Build history of the part. All positions in model axes, mm. Give positions to 0.01 mm unless a question says otherwise; leave off trailing zeros. Write each loop counter-clockwise with the first axis right and the second up, starting at its lowest first coordinate (ties: lowest second). Pieces come first, ordered by that corner, then holes. Notation, with made-up numbers: (30.5, 59) -> (85.5, 59) arc R21 ccw to (85.5, 71) -> close; hole circle Ø3 at (78.25, 39.5). An arc over 180 degrees is marked (long way). Put each result on its own line as item: value. Start each with the question number.
Item 1: Flat gauge pins, fed straight in: pin 1 Ø1.5 at (y, z) = (-53, 2) entering from -X; pin 2 Ø1 at (y, z) = (-55, 2) entering from -X. Where does each tip first touch, or does it go through?
Item 2: Slice it at B-B, the plane z = 2.3. List the corners of the cut face in (x, y).
Item 3: Slice it at C-C, the plane y = -68. List the corners of the cut face in (x, z).
Item 4: Drill centre lines: line 1 along X through (y, z) = (-64.5, 1.9); line 2 along X through (y, z) = (-65.5, 1.25); line 3 along Y through (x, z) = (70, 1.1). Where is each one in solid material? Low to high.
Item 5: Slice it at A-A, the plane x = 76. List the corners of the cut face in (y, z), plus the area to 3 significant figures.
Item 6: Slice it at D-D, the plane y = -35.5. List the corners of the cut face in (x, z), plus the area to 3 significant figures.
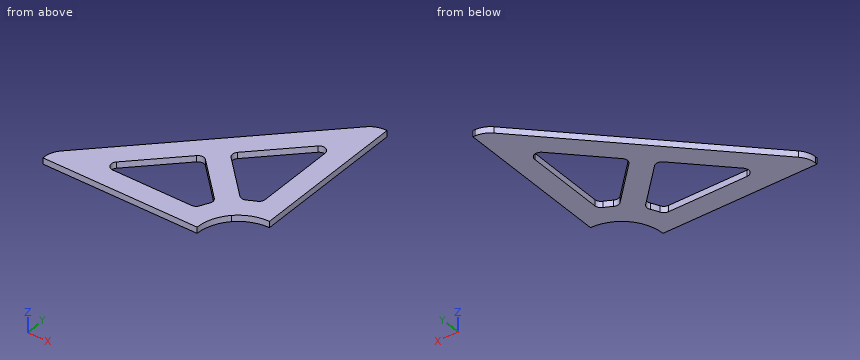
```python
from build123d import *

# Parameters (mm, degrees)
F1_DEPTH = 3
F2_R     = 3
F3_W     = 5
F3_H     = 3
F4_DEPTH = 25
F5_W     = 5
F5_H     = 3
F6_DEPTH = 25
F7_R     = 10


with BuildPart() as f1:
    # F0 (on Top) → F1 (new body)
    with BuildSketch(Plane.XY):
        with BuildLine():
            Line((50, -50), (0, -100))
            Line((0, -100), (70, -100))
            ThreePointArc((70, -100), (70.4320432104, -94.9269406382), (71.7157287525, -90))
            Line((71.7157287525, -90), (24.1421356237, -90))
            Line((24.1421356237, -90), (53.5355339059, -60.6066017178))
            Line((53.5355339059, -60.6066017178), (75.5479654307, -82.6190332426))
            ThreePointArc((75.5479654307, -82.6190332426), (77.0871215252, -80.635083269), (78.7867965644, -78.7867965644))
            Line((78.7867965644, -78.7867965644), (50, -50))
        make_face()
        with BuildLine():
            ThreePointArc((71.7157287525, -90), (70.4320432104, -94.9269406382), (70, -100))
            Line((70, -100), (80, -100))
            ThreePointArc((80, -100), (81.5224093498, -92.3463313527), (85.8578643763, -85.8578643763))
            Line((85.8578643763, -85.8578643763), (78.7867965644, -78.7867965644))
            ThreePointArc((78.7867965644, -78.7867965644), (77.0871215252, -80.635083269), (75.5479654307, -82.6190332426))
            ThreePointArc((75.5479654307, -82.6190332426), (73.3748398058, -86.1760770896), (71.7157287525, -90))
        make_face()
        with BuildLine():
            Line((100, -70), (100, 0))
            Line((100, 0), (50, -50))
            Line((50, -50), (78.7867965644, -78.7867965644))
            ThreePointArc((78.7867965644, -78.7867965644), (80.635083269, -77.0871215252), (82.6190332426, -75.5479654307))
            Line((82.6190332426, -75.5479654307), (60.6066017178, -53.5355339059))
            Line((60.6066017178, -53.5355339059), (90, -24.1421356237))
            Line((90, -24.1421356237), (90, -71.7157287525))
            ThreePointArc((90, -71.7157287525), (94.9269406382, -70.4320432104), (100, -70))
        make_face()
        with BuildLine():
            Line((100, -80), (100, -70))
            ThreePointArc((100, -70), (94.9269406382, -70.4320432104), (90, -71.7157287525))
            ThreePointArc((90, -71.7157287525), (86.1760770896, -73.3748398058), (82.6190332426, -75.5479654307))
            ThreePointArc((82.6190332426, -75.5479654307), (80.635083269, -77.0871215252), (78.7867965644, -78.7867965644))
            Line((78.7867965644, -78.7867965644), (85.8578643763, -85.8578643763))
            ThreePointArc((85.8578643763, -85.8578643763), (92.3463313527, -81.5224093498), (100, -80))
        make_face()
    extrude(amount=F1_DEPTH)

    # F2
    f2_edges = [f1.edges().sort_by_distance(p)[0] for p in [
        (24.142136, -90, 1.5),
        (53.535534, -60.606602, 1.5),
        (71.715729, -90, 1.5),
        (75.547965, -82.619033, 1.5),
        (60.606602, -53.535534, 1.5),
        (90, -71.715729, 1.5),
        (82.619033, -75.547965, 1.5),
        (90, -24.142136, 1.5),
    ]]
    fillet(f2_edges, radius=F2_R)

    # F3 (on face) → F4 (cut)
    with BuildSketch(Plane.XZ.offset(100)):
        with Locations((2.5, 1.5)):
            Rectangle(F3_W, F3_H)
    extrude(amount=-F4_DEPTH, mode=Mode.SUBTRACT)

    # F5 (on face) → F6 (cut)
    with BuildSketch(Plane.YZ.offset(100)):
        with Locations((-2.5, 1.5)):
            Rectangle(F5_W, F5_H)
    extrude(amount=-F6_DEPTH, mode=Mode.SUBTRACT)

    # F7
    f7_edges = [f1.edges().sort_by_distance(p)[0] for p in [
        (5, -95, 1.5),
        (95, -5, 1.5),
    ]]
    fillet(f7_edges, radius=F7_R)


solid = f1.part
```
Values follow:
1. pin 1: x = 46.25
1. pin 2: x = 44.5
2. outline: (5, -100) -> (80, -100) arc R20 cw to (100, -80) -> (100, -5) -> (99.14, -5) arc R10 ccw to (92.07, -7.93) -> (7.93, -92.07) arc R10 ccw to (5, -99.14) -> close; hole (29.26, -84.88) arc R3 ccw to (31.38, -90) -> (69.67, -90) arc R3 ccw to (72.43, -88.18) arc R30 cw to (74.28, -84.56) arc R3 ccw to (73.83, -80.9) -> (55.66, -62.73) arc R3 ccw to (51.41, -62.73) -> close; hole (62.73, -55.66) -> (80.9, -73.83) arc R3 ccw to (84.56, -74.28) arc R30 cw to (88.18, -72.43) arc R3 ccw to (90, -69.67) -> (90, -31.38) arc R3 ccw to (84.88, -29.26) -> (62.73, -51.41) arc R3 ccw to start
3. outline: (32, 0) -> (46.14, 0) -> (46.14, 3) -> (32, 3) -> close; (60.93, 0) -> (75.07, 0) -> (75.07, 3) -> (60.93, 3) -> close; (90, 0) -> (100, 0) -> (100, 3) -> (90, 3) -> close
4. line 1: 35.5 to 49.64, 57.43 to 71.57, 90 to 100
4. line 2: 34.5 to 48.64, 58.43 to 72.57, 90 to 100
4. line 3: -100 to -89.98, -77.07 to -62.93, -44.14 to -30
5. outline: (-100, 0) -> (-68.93, 0) -> (-68.93, 3) -> (-100, 3) -> close; (-38.14, 0) -> (-24, 0) -> (-24, 3) -> (-38.14, 3) -> close
5. area: 136 mm2
6. outline: (64.5, 0) -> (78.64, 0) -> (78.64, 3) -> (64.5, 3) -> close; (90, 0) -> (100, 0) -> (100, 3) -> (90, 3) -> close
6. area: 72.4 mm2
